The listing builds one solid part. Answer for the finished solid, in the listing's coordinates (mm). A direction names the side the tool comes from. Round coordinates to 2 decimals unless told otherwise and drop trailing zeros. Order: outer loops, then holes, each group sorted by start corner. A loop starts at its lowest first (then second) coordinate and runs counter-clockwise, first axis right, second up. Notation, with made-up numbers: (50.5, -24) - (107.5, -24) arc R6 ccw to (107.5, -14) - close; hole circle Ø5 at (-28.75, -34). An arc over 180 degrees is marked (long way). Write item = value, one per line.
Autodesk Inventor part; units mm, degrees
ref_plane "YZ Plane" through (0, 0, 0) normal (1, 0, 0) x (0, 1, 0)
ref_plane "XZ Plane" through (0, 0, 0) normal (0, 1, 0) x (-1, 0, 0)
ref_plane "XY Plane" through (0, 0, 0) normal (0, 0, 1) x (1, 0, 0)
sketch "Main Base Sketch" plane through (0, 0, 0) normal (0, 1, 0) x (-1, 0, 0)
  line L0 (75, -47) -> (75, 47)
  line L1 (-75, 47) -> (-75, -47)
  line L2 (-75, -47) -> (75, 47) construction
  line L3 (75, -47) -> (-75, 47) construction
  line L4 (-40, -47) -> (-40, -19)
  line L5 (-40, -19) -> (40, -19)
  line L6 (40, -19) -> (40, -47)
  line L7 (40, 19) -> (40, 47)
  line L8 (-40, 19) -> (40, 19)
  line L9 (-40, 47) -> (-40, 19)
  line L10 (75, 47) -> (40, 47)
  line L11 (-40, 47) -> (-75, 47)
  line L12 (-75, -47) -> (-40, -47)
  line L13 (40, -47) -> (75, -47)
  point P0 (0, 0)
  point P1 (0, 0)
  dimension "d0" = 94
  dimension "d1" = 35
  dimension "d2" = 35
  dimension "d3" = 80
  dimension "d4" = 150
  dimension "d5" = 28
  dimension "d6" = 94
  dimension "d8" = 80
  dimension "d9" = 28
  dimension "d27" = 28
  dimension "d28" = 38
  dimension "d37" = 0
extrude "Main Base Extrusion" add sketch "Main Base Sketch" along normal blind 6.5
sketch "Middle Cut Sketch" plane through (0, 6.5, 0) normal (0, 1, 0) x (1, 0, 0)
  line L0 (-75, 47) -> (-75, -47)
  line L1 (75, 19) -> (-75, 19)
  line L2 (-75, 19) -> (-75, -19)
  line L3 (-75, -19) -> (75, -19)
  line L4 (75, -19) -> (75, 19)
  line L5 (-40, -19) -> (40, -19)
  line L6 (75, -47) -> (75, 47)
  line L7 (40, 19) -> (-40, 19)
  point P0 (0, 0)
  dimension "d18" = 0
  dimension "d19" = 0
  dimension "d34" = 0
extrude "Middle Cut" cut sketch "Middle Cut Sketch" against normal blind 4.5
sketch "Arc Sketch" plane through (75, 0, 47) normal (1, 0, 0) x (0, 0, -1)
  line L0 (27, 9.9354) -> (27, -5.8008)
  line L1 (13.5, 9.3022) -> (13.5, -9.2521)
  line L2 (-4.6363, 2.5) -> (37.5698, 2.5)
  line L3 (94, 0) -> (0, 0) construction
  arc A0 (27, 2.5) -> (0, 2.5) centre (13.5, -18.2813) ccw
  line L4 (0, 8.4962) -> (0, -1.4448)
  line L5 (0, 0) -> (0, 6.5)
  line L6 (0, 6.5) -> (0, 2.5)
  line L7 (28, 6.5) -> (0, 6.5)
  line L8 (0, 6.5) -> (28, 6.5)
  line L9 (28, 2) -> (28, 6.5)
  line L10 (28, 6.5) -> (28, 2)
  line L11 (94, 0) -> (94, 6.5)
  line L12 (0, 6.5) -> (28, 6.5)
  line L13 (28, 2) -> (28, 6.5)
  line L14 (66, 2) -> (28, 2)
  line L15 (28, 2) -> (27, 2)
  line L16 (27, 2.5) -> (27, 2)
  dimension "d25" = 13.5
  dimension "d26" = 2.5
  dimension "d29" = 13.5
  dimension "d30" = 27
  dimension "d45" = 6.5
extrude "Arc Cut" cut sketch "Arc Sketch" against normal through all contours L2 L9 L15 L0 | A0 L7 L0 | L0 L7 L9 L2 | A0 L4 L7
mirror "Arc Mirror" about plane through (0, 0, 0) normal (0, 0, 1) of "Arc Cut"
sketch "Arc Holes Sketch" plane through (0, 0, 0) normal (0, -1, 0) x (1, 0, 0)
  circle A0 centre (57.5, 33.5) radius 2
  line L0 (75, -47) -> (75, 47)
  line L1 (40, 47) -> (40, 19)
  line L2 (40, 19) -> (-40, 19)
  line L3 (75, 47) -> (40, 47)
  line L4 (104.495, 0) -> (-129.4816, 0)
  line L5 (0, -57.7002) -> (0, 85.929)
  circle A1 centre (57.5, -33.5) radius 2
  circle A2 centre (-57.5, 33.5) radius 2
  circle A3 centre (-57.5, -33.5) radius 2
  point P0 (0, 0)
  dimension "d38" = 4
  dimension "d39" = 17.5
  dimension "d40" = 17.5
  dimension "d41" = 14.5
  dimension "d42" = 13.5
extrude "Arc Holes Cut" cut sketch "Arc Holes Sketch" against normal through all contours A0 | A1 | A2 | A3
properties part number "TapeMeasureBracketTop"
Q1. Section D-D on x = 42 is taken. Determine the outline of the cut face in (y, z).
Model answer:
outline = (0, -47) - (2.5, -47) arc R24.78 ccw to (2.5, -20) - (2, -20) - (2, 20) - (2.5, 20) arc R24.78 ccw to (2.5, 47) - (0, 47) - close
Q2. Section A-A on z = -33.5 is taken. Determine the outline of the cut face in (x, y).
Model answer:
outline = (-75, 0) - (-59.5, 0) - (-59.5, 6.5) - (-75, 6.5) - close; (-55.5, 0) - (-40, 0) - (-40, 6.5) - (-55.5, 6.5) - close; (40, 0) - (55.5, 0) - (55.5, 6.5) - (40, 6.5) - close; (59.5, 0) - (75, 0) - (75, 6.5) - (59.5, 6.5) - close
Q3. Determine the mould class of faces 1 (the face through (1, 0, 1)), 2 (the face through (-75, 1.8, -0.7)), 3 (the face through (40, 2, -33)) for opening direction X: released by +X, released by -X, zero draft, split by the parting line, or undercut.
Model answer:
face_1 = zero draft
face_2 = released by -X
face_3 = undercut
Q4. Section C-C on z = 29.5 is taken. Determine the outline of the cut face in (x, y).
Model answer:
outline = (-75, 0) - (-40, 0) - (-40, 6.18) - (-75, 6.18) - close; (40, 0) - (75, 0) - (75, 6.18) - (40, 6.18) - close
Q5. Flat-ended cylindrical pins translate along their axes: P1, Ø2, axis at x = 19.5, y = 1, coming from the +Z side; P2, Ø10, axis at x = -35.5, z = -16.5, coming from the -Y side; P3, Ø2, axis at x = 0, y = 1.5, coming from the -Z side. Find the tip coordinate at first contact, or state that the pin passes through.
Model answer:
P1 = 19
P2 = 0
P3 = -19
Q6. For faces 4 (the face through (-40, 2, -33)), 5 (the face through (58.423, 3.205, 31.726)), 6 (the face through (1, 2, 0)), 7 (the face through (75, 1.8, 0.7)), 8 (the face through (40, 2, 33)), determine the directions among +Z, -Z, +X, -X, +Y, -Y from which every point of the face is accessible in a straight line to the end or side of a thin tool.
Model answer:
face_4 = -Z, +Y, -Y
face_5 = +Y, -Y
face_6 = +X, -X, +Y
face_7 = +Z, -Z, +X, +Y, -Y
face_8 = +Z, +Y, -Y
Q7. Section B-B on y = 3.5 is taken. Determine the outline of the cut face in (x, z).
Model answer:
outline = (-75, -45.32) - (-40, -45.32) - (-40, -21.68) - (-75, -21.68) - close; (-75, 21.68) - (-40, 21.68) - (-40, 45.32) - (-75, 45.32) - close; (40, -45.32) - (75, -45.32) - (75, -21.68) - (40, -21.68) - close; (40, 21.68) - (75, 21.68) - (75, 45.32) - (40, 45.32) - close; hole circle Ø4 at (-57.5, -33.5); hole circle Ø4 at (-57.5, 33.5); hole circle Ø4 at (57.5, -33.5); hole circle Ø4 at (57.5, 33.5)
Q8. Find the intervals of material crossed by line 1 (X direction, y = 1.75, z = 33.5); line 2 (X direction, y = 0.5, z = -20); line 3 (Z direction, x = 57.5, y = 4.5), in increasing order. Write a range as from..to.
Model answer:
line_1 = -75..-59.5, -55.5..-40, 40..55.5, 59.5..75
line_2 = -75..-40, 40..75
line_3 = -43.25..-35.5, -31.5..-23.75, 23.75..31.5, 35.5..43.25
